The listing builds one solid part. Answer for the finished solid, in the listing's coordinates (mm). A direction names the side the tool comes from. Give positions to 0.01 mm unless a question says otherwise; leave off trailing zeros. Order: outer loops, then holes, each group sorted by start corner. A loop starts at its lowest first (then second) coordinate and runs counter-clockwise, first axis right, second up.
```python
from build123d import *

# Parameters (mm, degrees)
EXTRUDE_1_DEPTH = 35
SKETCH_2_R      = 5
EXTRUDE_2_DEPTH = 10


with BuildPart() as part:
    # 草图1 → 凸台-拉伸1 (new body)
    with BuildSketch(Plane(origin=(0, 0, 0), x_dir=(1, 0, 0), z_dir=(0, 1, 0))):
        Polygon((-23.5, 50), (-20, 60), (20, 60), (23.5, 50), (23.5, -50), (-23.5, -50), align=None)
    extrude(amount=EXTRUDE_1_DEPTH)

    # 草图2 → 凸台-拉伸2 (add)
    with BuildSketch(Plane(origin=(0, 35, 0), x_dir=(1, 0, 0), z_dir=(0, 1, 0))):
        with Locations(Location((-16.5, 55, 0), (0, 0, 90))):
            Circle(SKETCH_2_R)
        with Locations(Location((16.5, 55, 0), (0, 0, 90))):
            Circle(SKETCH_2_R)
    extrude(amount=EXTRUDE_2_DEPTH)


solid = part.part
```
1) Straight lines are drawn through the part: probe 1 along Y at (x, z) = (5, -19); probe 2 along X at (y, z) = (17.5, -53); probe 3 along Z at (x, y) = (13, 42). For each, find the intervals that lie inside material, in ascending order.
Geometry says:
probe 1: y = 0 to 35
probe 2: x = -22.45 to 22.45
probe 3: z = -58.57 to -51.43
2) Find section A-A (x = -13.5). Write down the section's boundary in (y, z), then the cut area to 3 significant figures.
Geometry says:
outline: (0, -60) - (35, -60) - (35, -59) - (45, -59) - (45, -51) - (35, -51) - (35, 50) - (0, 50) - close
area: 3,930 mm2
3) For a pull along X with two mould halves and no side action, classify faces 4 (the flat face through (23.5, 17, -1)), 5 (the cylindrical face through (-13.5, 39.9, -51)), 6 (the flat face through (16, 45, -55)) as +X half, -X half, draft (parallel to the pull), parting line (faces both ways), or undercut.
Geometry says:
face 4: +X half
face 5: undercut
face 6: draft
4) Find section D-D (x = -1). Write down the section's boundary in (y, z), then the cut area to 3 significant figures.
Geometry says:
outline: (0, -60) - (35, -60) - (35, 50) - (0, 50) - close
area: 3,850 mm2
5) Given P1, Ø10, axis at x = -5, y = 37, coming from the +Z side; P2, Ø10, axis at x = 1, z = 2.5, coming from the +Y side, each flat-ended and moving along its own axis, determine where each tip first touches the part or whether it passes through.
Geometry says:
P1: stops at z = 50
P2: stops at y = 35
6) Find section B-B (z = 43). Write down the section's boundary in (x, y), then the cut area to 4 significant figures.
Geometry says:
outline: (-23.5, 0) - (23.5, 0) - (23.5, 35) - (-23.5, 35) - close
area: 1,645 mm2
7) A tool of negligible diameter and unlimited length cuts with its end or side. For faces 1 (the cylindrical face through (19.5, 39.9, -51)), 2 (the flat face through (-20, 35, -59)), 3 (the flat face through (20, 35, -59)), from which of +Z, -Z, +X, -X, +Y, -Y can it reach the whole face along a straight path? Write none if from no direction.
Geometry says:
face 1: +Y
face 2: -Z, -X, +Y
face 3: -Z, +X, +Y
8) Find section C-C (x = 18.5). Write down the section's boundary in (y, z), then the cut area to 3 significant figures.
Geometry says:
outline: (0, -60) - (35, -60) - (35, -59.58) - (45, -59.58) - (45, -50.42) - (35, -50.42) - (35, 50) - (0, 50) - close
area: 3,940 mm2
